For this review, use the dimensioned drawing (mm, ordinates from the lowest corner) and the shaded views. Give positions to 0.01 mm unless a question says otherwise; leave off trailing zeros. Order: outer loops, then holes, each group sorted by start corner. A loop starts at its lowest first (then second) coordinate and runs counter-clockwise, first axis right, second up. Notation, with made-up numbers: M -21,-25 L 17,-25 A13 cw 17,-21 Z; hole C 28.25,-4 d3. An arc over 180 degrees is marked long. Answer as CSV lines item,"result". Start each with the question number.
1. We need section A-A, the plane z = 29. Give the boundary of the cut face in (x, y).
2. We need section C-C, the plane x = 56.75. Give the boundary of the cut face in (y, z), and give its area (3 significant figures).
3. Clearance check with flat-ended pins moving along their axes: P1, Ø2.5, axis at x = 7.25, z = 39, coming from the -Y side (1 decimal); P2, Ø3.5, axis at x = 4.5, z = 26, coming from the -Y side. State where each tip first meets the part, or that it passes through.
4. For line 1 along X through (y, z) = (1.4, 13); line 2 along X through (y, z) = (2.2, 29); line 3 along Z through (x, y) = (60, 0.45), list the stretches that pass through material, from the lowest coordinate up.
5. We need section B-B, the plane y = 0.9. State how many separate pieces and enclosed holes the cut face has, and give its area (3 significant figures).
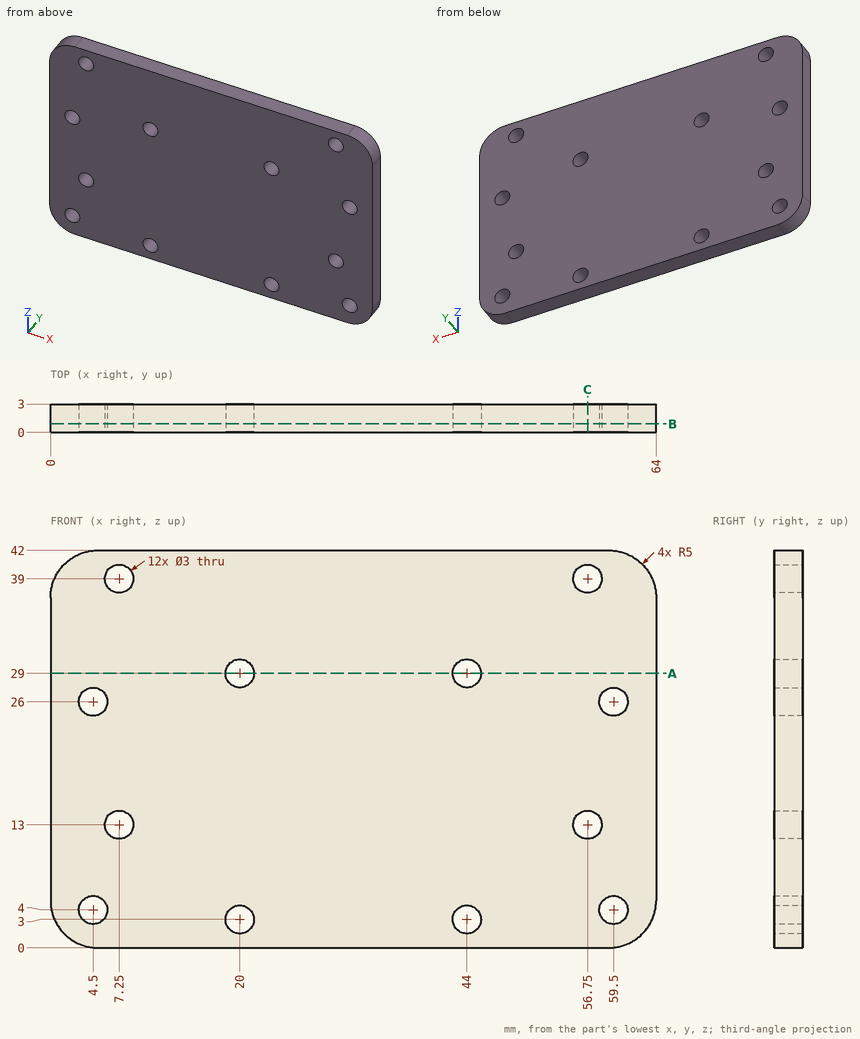
Result set:
1,outline,"M 0,0 L 18.5,0 L 18.5,3 L 0,3 Z; M 21.5,0 L 42.5,0 L 42.5,3 L 21.5,3 Z; M 45.5,0 L 64,0 L 64,3 L 45.5,3 Z"
2,outline,"M 0,0 L 3,0 L 3,11.5 L 0,11.5 Z; M 0,14.5 L 3,14.5 L 3,37.5 L 0,37.5 Z; M 0,40.5 L 3,40.5 L 3,42 L 0,42 Z"
2,area,"108 mm2"
3,P1,"through"
3,P2,"y = 0"
4,line 1,"0 to 5.75, 8.75 to 55.25, 58.25 to 64"
4,line 2,"0 to 18.5, 21.5 to 42.5, 45.5 to 64"
4,line 3,"0.1 to 2.59, 5.41 to 24.59, 27.41 to 41.9"
5,separate pieces,"1"
5,enclosed holes,"12"
5,area,"2,580 mm2"
